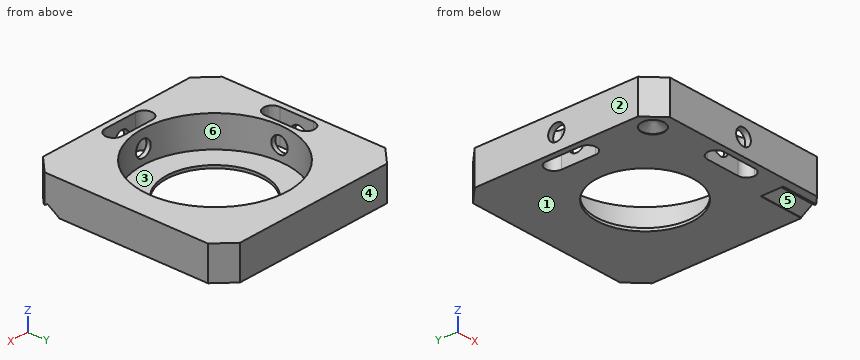
Autodesk Inventor part; units mm, degrees
ref_plane "YZ Plane" through (0, 0, 0) normal (1, 0, 0) x (0, 1, 0)
ref_plane "XZ Plane" through (0, 0, 0) normal (0, 1, 0) x (-1, 0, 0)
ref_plane "XY Plane" through (0, 0, 0) normal (0, 0, 1) x (1, 0, 0)
ref_plane "Work Plane1" through (0, 0, 2) normal (0, 0, 1) x (1, 0, 0)
sketch "Sketch1" plane through (0, 0, 2) normal (0, 0, 1) x (1, 0, 0)
  circle A0 centre (-37.0712, 14) radius 3.25 construction
  circle A1 centre (-9.0712, -14) radius 3.25 construction
  line L0 (-21.8762, -24.9) -> (-21.8762, -17.08) construction
  line L1 (-21.8762, -17.08) -> (-20.0712, -17.08) construction
  arc A2 (-20.0712, -17.08) -> (-20.0712, -14.08) centre (-20.0712, -15.58) ccw construction
  line L2 (-20.0712, -14.08) -> (-21.8762, -14.08) construction
  line L3 (-21.8762, -14.08) -> (-21.8762, -3.0223) construction
  arc A3 (-21.8762, -3.0223) -> (-25.9925, 1.4242) centre (-23.0712, 0) ccw construction
  line L4 (-25.9925, 1.4242) -> (-37.0712, 1.4242) construction
  line L5 (-37.0712, 1.4242) -> (-37.0712, 3) construction
  arc A4 (-37.0712, 3) -> (-40.0712, 3) centre (-38.5712, 3) ccw construction
  line L6 (-40.0712, 3) -> (-40.0712, 1.4242) construction
  line L7 (-40.0712, 1.4242) -> (-47.9712, 1.4242) construction
  line L8 (-47.9712, 1.4242) -> (-47.9712, 17) construction
  line L9 (-47.9712, 17) -> (-44.3964, 17) construction
  line L10 (-44.3964, 17) -> (-40.0712, 21.3252) construction
  line L11 (-40.0712, 21.3252) -> (-40.0712, 24.9) construction
  line L12 (-40.0712, 24.9) -> (-6.0712, 24.9) construction
  line L13 (-6.0712, 24.9) -> (-6.0712, 21.3252) construction
  line L14 (-6.0712, 21.3252) -> (-1.746, 17) construction
  line L15 (-1.746, 17) -> (1.8288, 17) construction
  line L16 (1.8288, 17) -> (1.8288, -17) construction
  line L17 (1.8288, -17) -> (-1.746, -17) construction
  line L18 (-1.746, -17) -> (-6.1126, -21.3666) construction
  line L19 (-6.1126, -21.3666) -> (-6.1126, -24.9) construction
  line L20 (-6.1126, -24.9) -> (-21.8762, -24.9) construction
  circle A5 centre (-37.0712, -14) radius 3.25 construction
  circle A6 centre (-23.0712, 0) radius 12.45 construction
  circle A7 centre (-23.0712, 0) radius 12.7 construction
  line L21 (-37.0712, 14) -> (-9.0712, 14) construction
  line L22 (-9.0712, 14) -> (-9.0712, -14) construction
  line L23 (-9.0712, -14) -> (-37.0712, -14) construction
  line L24 (-37.0712, -14) -> (-37.0712, 14) construction
  line L25 (-5.5712, -17.5) -> (-5.5712, 17.5)
  line L26 (-5.5712, 17.5) -> (-40.5712, 17.5)
  line L27 (-40.5712, 17.5) -> (-40.5712, -17.5)
  line L28 (-40.5712, -17.5) -> (-5.5712, -17.5)
  circle A8 centre (-23.0712, 0) radius 12.8
  point P0 (0, 0)
  dimension "d0" = 3.5
  dimension "d1" = 0.1
extrude "Extrusion1" add sketch "Sketch1" along normal blind 6
sketch "Sketch2" plane through (0, 0, 2) normal (0, 0, -1) x (-1, 0, 0)
  circle A0 centre (23.0712, 0) radius 12.8
  circle A1 centre (23.0712, 0) radius 8.5824
  line L0 (5.5712, -17.5) -> (5.5712, 17.5)
  line L1 (5.5712, 17.5) -> (40.5712, 17.5)
  point P0 (0, 0)
  point P1 (5.5712, 0)
  point P2 (23.0712, 17.5)
  point P3 (5.5712, 0)
  point P4 (5.5712, 0)
  point P5 (5.5712, 0)
  point P6 (23.0712, 17.5)
  point P7 (23.0712, 17.5)
  point P8 (23.0712, 17.5)
extrude "Extrusion2" add sketch "Sketch2" against normal blind 0.5
sketch "Sketch3" plane through (0, 0, 2) normal (0, 0, -1) x (-1, 0, 0)
  circle A0 centre (9.0712, -14) radius 1.45 construction
  circle A1 centre (9.0712, -14) radius 2.45
  circle A2 centre (37.0712, -14) radius 1.45
  circle A3 centre (37.0712, -14) radius 1.95
  point P0 (0, 0)
  dimension "d8" = 1
  dimension "d10" = 0.5
sketch "Sketch5" plane through (0, 0, 2) normal (0, 0, -1) x (-1, 0, 0)
  arc A0 (20.0712, -14.08) -> (20.0712, -17.08) centre (20.0712, -15.58) ccw
  arc A1 (26.0712, -17.08) -> (26.0712, -14.08) centre (26.0712, -15.58) ccw
  line L0 (37.0712, 3) -> (37.0712, -3)
  arc A2 (37.0712, -3) -> (40.0712, -3) centre (38.5712, -3) ccw
  line L1 (40.0712, -3) -> (40.0712, 3)
  arc A3 (40.0712, 3) -> (37.0712, 3) centre (38.5712, 3) ccw
  line L2 (26.0712, -14.08) -> (20.0712, -14.08)
  arc A4 (20.0712, -14.08) -> (20.0712, -17.08) centre (20.0712, -15.58) ccw
  line L3 (20.0712, -17.08) -> (26.0712, -17.08)
  arc A5 (26.0712, -17.08) -> (26.0712, -14.08) centre (26.0712, -15.58) ccw
  circle A6 centre (37.0712, -14) radius 1.45
  circle A7 centre (23.0712, 0) radius 1.45
  circle A8 centre (9.0712, -14) radius 1.45
  circle A9 centre (37.0712, 14) radius 1.45
  line L4 (-1.8288, -17) -> (-1.8288, 17)
  line L5 (-1.8288, 17) -> (1.746, 17)
  line L6 (1.746, 17) -> (6.0712, 21.3252)
  line L7 (6.0712, 21.3252) -> (6.0712, 24.9)
  line L8 (6.0712, 24.9) -> (40.0712, 24.9)
  line L9 (40.0712, 24.9) -> (40.0712, 21.3252)
  line L10 (40.0712, 21.3252) -> (44.3964, 17)
  line L11 (44.3964, 17) -> (47.9712, 17)
  line L12 (47.9712, 17) -> (47.9712, -17)
  line L13 (44.3964, -17) -> (47.9712, -17)
  line L14 (40.0712, -21.3252) -> (44.3964, -17)
  line L15 (40.0712, -24.9) -> (40.0712, -21.3252)
  line L16 (6.1126, -24.9) -> (40.0712, -24.9)
  line L17 (6.1126, -24.9) -> (6.1126, -21.3666)
  line L18 (6.1126, -21.3666) -> (1.746, -17)
  line L19 (1.746, -17) -> (-1.8288, -17)
  line L20 (40.5712, -17.5) -> (5.5712, -17.5)
  arc A10 (19.7251, -13.5) -> (18.2262, -15.0577) centre (19.7251, -15) ccw
  arc A11 (25.7274, -16.5) -> (25.7274, -16.5) centre (25.7274, -15) ccw
  line L21 (25.7274, -13.5) -> (25.7274, -13.5)
  arc A12 (19.7251, -13.5) -> (18.2262, -15.0577) centre (19.7251, -15) ccw
  line L22 (19.7251, -16.5) -> (19.7251, -16.5)
  arc A13 (25.7274, -16.5) -> (25.7274, -16.5) centre (25.7274, -15) ccw
  arc A14 (18.3936, -15.6908) -> (19.7251, -16.5) centre (19.7251, -15) ccw
  arc A15 (18.2262, -15.0577) -> (18.3936, -15.6908) centre (19.7251, -15) ccw
  arc A16 (18.3936, -15.6908) -> (19.7251, -16.5) centre (19.7251, -15) ccw
  arc A17 (18.2262, -15.0577) -> (18.3936, -15.6908) centre (19.7251, -15) ccw
  arc A18 (26.9396, -15.8835) -> (27.2262, -15.0582) centre (25.7274, -15) ccw
  arc A19 (26.9396, -15.8835) -> (27.2262, -15.0582) centre (25.7274, -15) ccw
  arc A20 (27.2262, -15.0582) -> (25.7274, -13.5) centre (25.7274, -15) ccw
  arc A21 (27.2262, -15.0582) -> (25.7274, -13.5) centre (25.7274, -15) ccw
  line L23 (19.7251, -16.5) -> (25.7274, -16.5)
  line L24 (25.7274, -13.5) -> (19.7251, -13.5)
  line L25 (19.7251, -13.5) -> (19.7251, -13.5)
  arc A22 (25.7274, -16.5) -> (26.9396, -15.8835) centre (25.7274, -15) ccw
  arc A23 (25.7274, -16.5) -> (26.9396, -15.8835) centre (25.7274, -15) ccw
  point P0 (0, 0)
  point P1 (40.0712, -3)
  point P2 (22.6287, -9.823)
  point P3 (22.6523, -12.823)
  point P4 (19.7251, -16.5)
  point P5 (25.7274, -16.5)
  point P6 (25.7274, -13.5)
  point P7 (19.7251, -13.5)
  dimension "d50" = 9
  dimension "d52" = 3
  dimension "d53" = 1.5
  dimension "d56" = 1.5
  dimension "d57" = 1.5
  dimension "d58" = 1.5
  dimension "d59" = 1
extrude "Extrusion5" cut sketch "Sketch5" against normal blind 8 contours L2 A11 L23 A14 A0 | A0 A14 A15 A10 L24 A11 L2 | A11 A1 L2 | L2 A1 A11
sketch "Sketch6" plane through (-40.5712, -17.5, 8) normal (0, -1, 0) x (1, 0, 0)
  line L0 (0, -6) -> (35, -6)
  line L1 (35, -6) -> (35, 0)
  line L2 (0, 0) -> (35, 0)
  line L3 (0, -6) -> (0, 0)
  line L4 (30.3, 0) -> (30.3, 0)
  circle A0 centre (17.5, -3) radius 1.45
  point P0 (40.5712, -8)
  point P1 (17.5, 0)
  point P2 (35, -3)
  dimension "d34" = 2.9
extrude "Extrusion6" cut sketch "Sketch6" against normal blind 8 contours A0
pattern_circular "Circular Pattern1" count 2 over 90 about axis through (-23.0712, 0, 2) along (0, 0, -1) of "Extrusion6"
chamfer "Chamfer1" distance 3 angle 45 4 edges at (-40.5712, 17.5, 5) (-5.5712, 17.5, 5) (-5.5712, -17.5, 5) (-40.5712, -17.5, 5)
hole "Hole1" at (-37.0712, -14, 2) direction (0, 0, 1) diameter 4 depth 0.1 tip angle 115
sketch "Sketch4" plane through (-5.5712, -17.5, 2) normal (1, 0, 0) x (0, 0, -1)
  line L0 (2, 4.45) -> (6, 4.45)
  line L1 (2, 1.55) -> (6, 1.55)
  line L2 (0, 0) -> (0, 35)
  arc A0 (2, 19) -> (2, 19) centre (1.5, 4.4206) ccw
  line L3 (-1.3741, 3.5) -> (-0.1, 5.5)
  line L4 (-1.3741, 3.5) -> (-0.1, 1.5)
  line L5 (-0.1, 5.5) -> (0.6045, 5.5)
  line L6 (0.6045, 5.5) -> (0.6045, 1.5)
  line L7 (0.6045, 1.5) -> (-0.1, 1.5)
  line L8 (-0.1, 1.5) -> (-0.1, 5.5)
  point P0 (2, 17.5)
  point P1 (-0.1, 1.5)
extrude "Extrusion4" cut sketch "Sketch4" against normal blind 8 contours L7 L8 L5 L2 | L2 L5 L6 L7 | L4 L3 L8
pattern_circular "Circular Pattern2" count 2 over 90 about axis through (-23.0712, 0, 2) along (0, 0, -1) of "Extrusion5"
equation "\"d50\" = d49"
equation "\"d52\" = d51"
equation "\"d53\" = d55"
equation "\"d56\" = d55"
properties part number "20_Cube_Insert_Kinematic_KES400AMount_45_UPD_v3"
The listing builds one solid part. Answer for the finished solid, in the listing's coordinates (mm). Face numbers are marked on the shaded views. A direction names the side the tool comes from. Round coordinates to 2 decimals unless told otherwise and drop trailing zeros. Write each loop counter-clockwise with the first axis right and the second up, starting at its lowest first coordinate (ties: lowest second). Pieces come first, ordered by that corner, then holes. Notation, with made-up numbers: (21, 74) - (59, 74) arc R21 ccw to (59, 93) - close; hole circle Ø8 at (55, 43). An arc over 180 degrees is marked (long way). Use a Markdown table: item, result. Add a question column.
1. The part is cut by section C-C (y = 15.5). Write down the section's boundary in (x, z).
2. Consider line 1 (Y direction, x = -23, z = 7); line 2 (X direction, y = 3, z = 4.75); line 3 (X direction, y = 1, z = 3.75). Determine where each line is inside the solid, lowest interval first.
3. The part is cut by section A-A (z = 7.5). Write down the section's boundary in (x, y) (3 decimals).
4. The part is cut by section B-B (y = 0). Write down the section's boundary in (x, z).
5. For a pull along X with two mould halves and no side action, classify the marked faces 1, 2 and 3 as +X half, -X half, draft (parallel to the pull), parting line (faces both ways), or undercut.
6. A tool of negligible diameter and unlimited length cuts with its end or side. For the marked faces 4, 5 and 6, from which of +Z, -Z, +X, -X, +Y, -Y can it reach the whole face along a straight path? Write none if from no direction.
Reported:
| question | item | result |
|---|---|---|
| 1 | outline | (-39.57, 2) - (-6.57, 2) - (-6.57, 8) - (-39.57, 8) - close |
| 2 | line 1 | -17.5 to -16.5, -13.5 to -12.8, 12.8 to 17.5 |
| 2 | line 2 | -40.57 to -39.53, -36.61 to -35.51, -10.63 to -5.57 |
| 2 | line 3 | -40.57 to -39.57, -36.57 to -35.83, -10.31 to -5.57 |
| 3 | outline | (-40.571, -14.5) - (-37.571, -17.5) - (-8.571, -17.5) - (-5.571, -14.5) - (-5.571, 14.5) - (-8.571, 17.5) - (-37.571, 17.5) - (-40.571, 14.5) - close; hole (-39.571, -3.346) arc R1.5 ccw to (-38.762, -4.678) arc R1.5 ccw to (-38.129, -4.845) arc R1.5 ccw to (-36.571, -3.346) - (-36.571, 2.656) arc R1.5 ccw to (-39.571, 2.656) - close; hole circle Ø25.6 at (-23.071, 0); hole (-25.727, -16.5) - (-19.725, -16.5) arc R1.5 ccw to (-18.394, -15.691) arc R1.5 ccw to (-18.226, -15.058) arc R1.5 ccw to (-19.725, -13.5) - (-25.727, -13.5) arc R1.5 ccw to start |
| 4 | outline | (-40.57, 2) - (-39.57, 2) - (-39.57, 3.55) - (-40.57, 3.55) - close; (-40.57, 6.45) - (-39.57, 6.45) - (-39.57, 8) - (-40.57, 8) - close; (-36.57, 2) - (-31.65, 2) - (-31.65, 2.5) - (-35.87, 2.5) - (-35.87, 3.55) - (-36.57, 3.55) - close; (-36.57, 6.45) - (-35.87, 6.45) - (-35.87, 8) - (-36.57, 8) - close; (-14.49, 2) - (-5.57, 2) - (-5.57, 8) - (-10.27, 8) - (-10.27, 2.5) - (-14.49, 2.5) - close |
| 5 | face 1 | draft |
| 5 | face 2 | -X half |
| 5 | face 3 | undercut |
| 6 | face 4 | +Z, -Z, +X, -X, +Y |
| 6 | face 5 | -Z, +X |
| 6 | face 6 | +Z |
